from build123d import *

# Parameters (mm, degrees)
F0_W     = 25.2
F0_H     = 24
F0_R     = 1
F3_DEPTH = 1
F4_DEPTH = 3.5
F5_DEPTH = 5.3
F2_W     = 21.4
F2_H     = 5.7
F6_DEPTH = 3.75


with BuildPart() as f3:
    # F0 (on Front) → F3 (new body)
    with BuildSketch(Plane.XZ):
        Rectangle(F0_W, F0_H)
        with Locations((-10.6, -2.6)):
            Circle(F0_R, mode=Mode.SUBTRACT)
        with Locations((10.6, -2.6)):
            Circle(F0_R, mode=Mode.SUBTRACT)
        with Locations((-10.6, 10)):
            Circle(F0_R, mode=Mode.SUBTRACT)
        with Locations((10.6, 10)):
            Circle(F0_R, mode=Mode.SUBTRACT)
    extrude(amount=-F3_DEPTH)

    # F1 (on face) → F4 (join)
    with BuildSketch(Plane.XZ):
        with BuildLine():
            Line((0, -6.6), (4, -6.6))
            Line((4, -6.6), (4, -2.6))
            ThreePointArc((4, -2.6), (2.828427, -5.428427), (0, -6.6))
        make_face()
        with BuildLine():
            Line((-4, -6.6), (0, -6.6))
            ThreePointArc((0, -6.6), (-2.828427, -5.428427), (-4, -2.6))
            Line((-4, -2.6), (-4, -6.6))
        make_face()
        with BuildLine():
            ThreePointArc((0, 1.4), (2.828427, 0.228427), (4, -2.6))
            Line((4, -2.6), (4, 1.4))
            Line((4, 1.4), (0, 1.4))
        make_face()
        with BuildLine():
            Line((-4, 1.4), (-4, -2.6))
            ThreePointArc((-4, -2.6), (-2.828427, 0.228427), (0, 1.4))
            Line((0, 1.4), (-4, 1.4))
        make_face()
    extrude(amount=F4_DEPTH)

    # F1 (on face) → F5 (join)
    with BuildSketch(Plane.XZ):
        with BuildLine():
            ThreePointArc((-4, -2.6), (-2.828427, -5.428427), (0, -6.6))
            ThreePointArc((0, -6.6), (2.828427, -5.428427), (4, -2.6))
            ThreePointArc((4, -2.6), (2.828427, 0.228427), (0, 1.4))
            ThreePointArc((0, 1.4), (-2.828427, 0.228427), (-4, -2.6))
        make_face()
    extrude(amount=F5_DEPTH)

    # F2 (on face) → F6 (join)
    with BuildSketch(Plane.XZ):
        with Locations((0, -9.15)):
            Rectangle(F2_W, F2_H)
    extrude(amount=-F6_DEPTH)


solid = f3.part
The model under review builds one solid part; all positions refer to its coordinate system, in mm. A direction names the side the tool comes from. Round coordinates to 2 decimals unless told otherwise and drop trailing zeros. Loops run counter-clockwise (first coordinate to the right, second up) from the corner with the lowest first, then second, coordinate; pieces in that order, holes last. Notation, with made-up numbers: (47.5, 88.5) -> (64.5, 88.5) arc R20 cw to (64.5, 125.5) -> close; hole circle Ø8 at (-4, 1). An arc over 180 degrees is marked (long way). Return JSON: item names as keys, results as strings.
(1) The part is to be moulded in two halves that separate along Z. For faces 1 (the flat face through (0, -2, 1.4)), 2 (the flat face through (0, -2, -6.6)), 3 (the cylindrical face through (-11.6, 0.5, -2.6)), 4 (the flat face through (0, 1, 3)), say which applies: released by +Z, released by -Z, zero draft, split by the parting line, or undercut.
Solved:
{"face 1": "released by +Z", "face 2": "released by -Z", "face 3": "undercut", "face 4": "zero draft"}
(2) Add section C-C on x = 6.75. Write out the cut boundary in (y, z).
Solved:
{"outline": "(0, -12) -> (3.75, -12) -> (3.75, -6.3) -> (1, -6.3) -> (1, 12) -> (0, 12) -> close"}
(3) For pin 1 (4 mm diameter, centred on x = 5, z = 3.5, fed in from -Y); pin 2 (6 mm diameter, centred on x = -4.5, z = 1.5, fed in from +Y); pin 3 (1 mm diameter, centred on y = 2.5, z = -8, fed in from +X), all flat-tipped, find the tip position at first contact; note any pin that passes through.
Solved:
{"pin 1": "y = 0", "pin 2": "y = 1", "pin 3": "x = 10.7"}
(4) For line 1 (Z direction, x = -10.6, y = 0.45); line 2 (X direction, y = 0.75, z = -2); line 3 (Y direction, x = -1.25, z = 3.75), list the stretches that pass through material, from the lowest coordinate up.
Solved:
{"line 1": "-12 to -3.6, -1.6 to 9, 11 to 12", "line 2": "-12.6 to -11.4, -9.8 to 9.8, 11.4 to 12.6", "line 3": "0 to 1"}
(5) For faces 5 (the flat face through (-3, -3.5, -6)), 6 (the flat face through (3, -3.5, 1)), 7 (the flat face through (-4, -2, -3)), 8 (the flat face through (-3.2, -3.5, 0.4)), list the 3-axis set-ups (+Z, -Z, +X, -X, +Y, -Y) from which the entire face can be reached by the end or side of a thin tool; tool diameter is ignored.
Solved:
{"face 5": "-Z, -X, -Y", "face 6": "+Z, +X, -Y", "face 7": "+Z, -Z, -X, -Y", "face 8": "+Z, -X, -Y"}
(6) Add section A-A on z = 10. Write out the cut boundary in (x, y).
Solved:
{"outline": "(-12.6, 0) -> (-11.6, 0) -> (-11.6, 1) -> (-12.6, 1) -> close; (-9.6, 0) -> (9.6, 0) -> (9.6, 1) -> (-9.6, 1) -> close; (11.6, 0) -> (12.6, 0) -> (12.6, 1) -> (11.6, 1) -> close"}
(7) Add section D-D on y = 2. Write out the cut boundary in (x, z).
Solved:
{"outline": "(-10.7, -12) -> (10.7, -12) -> (10.7, -6.3) -> (-10.7, -6.3) -> close"}
(8) Add section B-B on z = -10.5. Write out the cut boundary in (x, y).
Solved:
{"outline": "(-12.6, 0) -> (12.6, 0) -> (12.6, 1) -> (10.7, 1) -> (10.7, 3.75) -> (-10.7, 3.75) -> (-10.7, 1) -> (-12.6, 1) -> close"}
